```python
from build123d import *

# Parameters (mm, degrees)
PCB_DEPTH           = 1.56
ESQUISSE2_W         = 6
ESQUISSE2_H         = 6
ESQUISSE2_R         = 1.75
CORPSBP_DEPTH       = 3.52
ESQUISSE2_3_R       = 1.75
BPBP_DEPTH          = 4.32
ESQUISSE2_4_W       = 3.54
ESQUISSE2_4_H       = 8.6
CORPSONOFF_DEPTH    = 3.5
ESQUISSE2_5_W       = 1.5
ESQUISSE2_5_H       = 3.6
BPONOFF_DEPTH       = 5.5
ESQUISSE2_6_W       = 5
ESQUISSE2_6_H       = 5
BOSS_EXTRU_9_DEPTH  = 1.5
ESQUISSE5_R         = 5.9
BUZZER_DEPTH        = 9.9
ESQUISSE5_4_W       = 7.74
ESQUISSE5_4_H       = 5
ISP_DEPTH           = 8.6
CR2032_DEPTH        = 7
ESQUISSE6_W         = 4
ESQUISSE6_H         = 4
BOSS_EXTRU_10_DEPTH = 1.5


with BuildPart() as part:
    # Esquisse1 → PCB (new body)
    with BuildSketch(Plane.XY):
        with BuildLine():
            Line((-25.15, -25.15), (25.15, -25.15))
            ThreePointArc((25.15, -25.15), (28.685533906, -23.685533906), (30.15, -20.15))
            Line((30.15, -20.15), (30.15, 20.15))
            ThreePointArc((30.15, 20.15), (28.685533906, 23.685533906), (25.15, 25.15))
            Line((25.15, 25.15), (-25.15, 25.15))
            ThreePointArc((-25.15, 25.15), (-28.685533906, 23.685533906), (-30.15, 20.15))
            Line((-30.15, 20.15), (-30.15, -20.15))
            ThreePointArc((-30.15, -20.15), (-28.685533906, -23.685533906), (-25.15, -25.15))
        make_face()
    extrude(amount=PCB_DEPTH)

    # Esquisse2 → CorpsBp (add)
    # profile 1 of 8: a face of its own
    with BuildSketch(Plane.XY.offset(1.56)):
        with Locations((-20.15, 9.75)):
            Rectangle(ESQUISSE2_W, ESQUISSE2_H)
        with Locations((-20.15, 9.75)):
            Circle(ESQUISSE2_R, mode=Mode.SUBTRACT)
    # profile 2 of 8: a face of its own
    with BuildSketch(Plane.XY.offset(1.56)):
        with Locations((-20.45, -10.35)):
            Rectangle(ESQUISSE2_W, ESQUISSE2_H)
        with Locations((-20.45, -10.35)):
            Circle(ESQUISSE2_R, mode=Mode.SUBTRACT)
    # profile 3 of 8: a face of its own
    with BuildSketch(Plane.XY.offset(1.56)):
        with Locations((20.31, 9.55)):
            Rectangle(ESQUISSE2_W, ESQUISSE2_H)
        with Locations((20.31, 9.55)):
            Circle(ESQUISSE2_R, mode=Mode.SUBTRACT)
    # profile 4 of 8: a face of its own
    with BuildSketch(Plane.XY.offset(1.56)):
        with Locations((19.85, -10.35)):
            Rectangle(ESQUISSE2_W, ESQUISSE2_H)
        with Locations((19.85, -10.35)):
            Circle(ESQUISSE2_R, mode=Mode.SUBTRACT)
    # profile 5 of 8: a face of its own
    with BuildSketch(Plane.XY.offset(1.56)):
        with Locations((-20.45, -10.35)):
            Circle(ESQUISSE2_R)
    # profile 6 of 8: a face of its own
    with BuildSketch(Plane.XY.offset(1.56)):
        with Locations((-20.15, 9.75)):
            Circle(ESQUISSE2_R)
    # profile 7 of 8: a face of its own
    with BuildSketch(Plane.XY.offset(1.56)):
        with Locations((20.31, 9.55)):
            Circle(ESQUISSE2_R)
    # profile 8 of 8: a face of its own
    with BuildSketch(Plane.XY.offset(1.56)):
        with Locations((19.85, -10.35)):
            Circle(ESQUISSE2_R)
    extrude(amount=CORPSBP_DEPTH)

    # Esquisse2_3 → BpBp (add)
    with BuildSketch(Plane.XY.offset(1.56)):
        with Locations((20.31, 9.55)):
            Circle(ESQUISSE2_3_R)
        with Locations((-20.15, 9.75)):
            Circle(ESQUISSE2_3_R)
        with Locations((-20.45, -10.35)):
            Circle(ESQUISSE2_3_R)
        with Locations((19.85, -10.35)):
            Circle(ESQUISSE2_3_R)
    extrude(amount=BPBP_DEPTH)

    # Esquisse2_4 → CorpsOnOff (add)
    with BuildSketch(Plane.XY.offset(1.56)):
        with Locations((9.04, 9.85)):
            Rectangle(ESQUISSE2_4_W, ESQUISSE2_4_H)
    extrude(amount=CORPSONOFF_DEPTH)

    # Esquisse2_5 → BpOnOff (add)
    with BuildSketch(Plane.XY.offset(1.56)):
        with Locations((9.04, 9.85)):
            Rectangle(ESQUISSE2_5_W, ESQUISSE2_5_H)
    extrude(amount=BPONOFF_DEPTH)

    # Esquisse2_6 → Boss.-Extru.9 (add)
    with BuildSketch(Plane.XY.offset(1.56)):
        with Locations((-12.5, 17.5)):
            Rectangle(ESQUISSE2_6_W, ESQUISSE2_6_H)
        with Locations((-12.5, -17.5)):
            Rectangle(ESQUISSE2_6_W, ESQUISSE2_6_H)
        with Locations((12.5, -17.5)):
            Rectangle(ESQUISSE2_6_W, ESQUISSE2_6_H)
        with Locations((12.5, 17.5)):
            Rectangle(ESQUISSE2_6_W, ESQUISSE2_6_H)
    extrude(amount=BOSS_EXTRU_9_DEPTH)

    # Esquisse5 → Buzzer (add)
    with BuildSketch(Plane(origin=(0, 0, 0), x_dir=(-1, 0, 0), z_dir=(0, 0, -1))):
        with Locations(Location((0.75, -18.69, 0), (0, 0, 180))):
            Circle(ESQUISSE5_R)
    extrude(amount=BUZZER_DEPTH)

    # Esquisse5_4 → ISP (add)
    with BuildSketch(Plane(origin=(0, 0, 0), x_dir=(-1, 0, 0), z_dir=(0, 0, -1))):
        with Locations((0, 16.45)):
            Rectangle(ESQUISSE5_4_W, ESQUISSE5_4_H)
    extrude(amount=ISP_DEPTH)

    # Esquisse5_5 → CR2032 (add)
    with BuildSketch(Plane(origin=(0, 0, 0), x_dir=(-1, 0, 0), z_dir=(0, 0, -1))):
        with BuildLine():
            Line((9.061920088, 3.25), (15.15, 3.25))
            Line((15.15, 3.25), (15.15, -3.35))
            Line((15.15, -3.35), (9.061920088, -3.35))
            ThreePointArc((9.061920088, -3.35), (-13.25, -0.05), (9.061920088, 3.25))
        make_face()
    extrude(amount=CR2032_DEPTH)

    # Esquisse6 → Boss.-Extru.10 (add)
    with BuildSketch(Plane.XY.offset(1.56)):
        with Locations((-24.35, -17.8)):
            Rectangle(ESQUISSE6_W, ESQUISSE6_H)
    extrude(amount=BOSS_EXTRU_10_DEPTH)


solid = part.part
```
CAD build for the part. Positions are in the model's coordinates, mm. A direction names the side the tool comes from. Round coordinates to 2 decimals unless told otherwise and drop trailing zeros. Write each loop counter-clockwise with the first axis right and the second up, starting at its lowest first coordinate (ties: lowest second). Pieces come first, ordered by that corner, then holes. Notation, with made-up numbers: (-36, 83.25) - (23, 83.25) arc R25 ccw to (23, 106.25) - close; hole circle Ø10 at (88.5, -31.75). An arc over 180 degrees is marked (long way). Return JSON: item names as keys, results as strings. Group by question number.
Item 1: Band-saw the part on B-B on z = -6. List the corners of the cut face in (x, y).
Item 2: Band-saw the part on A-A on x = -11.5. List the corners of the cut face in (y, z).
Item 3: Band-saw the part on C-C on y = -18.69. List the corners of the cut face in (x, z).
Item 4: Probe probe 1 along Y at (x, z) = (-10.5, 2.75); probe 2 along X at (y, z) = (-15.5, 2.25); probe 3 along Z at (x, y) = (4, -2). List the from-to ranges inside material, lowest first.
Item 5: Flat gauge pins, fed straight in: pin 1 Ø3 at (x, y) = (-19.5, 10.5) entering from +Z; pin 2 Ø0.6 at (y, z) = (10, 6.5) entering from -X; pin 3 Ø8 at (y, z) = (16, 4) entering from +X; pin 4 Ø1 at (x, y) = (-9, 19) entering from -Z. Where does each tip first touch, or does it go through?
Item 6: 3-axis set-ups, long thin cutter, end or side, ignore diameter. For faces 1 (the face through (12, 15, 2)), 2 (the face through (10, 17, 2)), 3 (the face through (12, 18, 3.06)), 4 (the face through (-26.35, -18, 2)): which of +Z, -Z, +X, -X, +Y, -Y reach the whole face in a straight line?
Item 7: Band-saw the part on D-D on y = 18. List the corners of the cut face in (x, z), plus the area to 3 significant figures.
Item 8: Mould opens along Y. For faces 5 (the face through (21, -12, 5.08)), 6 (the face through (10, 10, 5.06)), 7 (the face through (28.65, -23.72, 0.77)) say: +Y half, -Y half, draft (parallel to the pull), parting line (faces both ways), or undercut.
Resolved:
{
 "1": {"outline": "(-15.15, -3.35) - (-9.06, -3.35) arc R11.4 ccw (long way) to (-9.06, 3.25) - (-15.15, 3.25) - close; circle Ø11.8 at (-0.75, -18.69); (-3.87, 13.95) - (3.87, 13.95) - (3.87, 18.95) - (-3.87, 18.95) - close"},
 "2": {"outline": "(-25.15, 0) - (-3.35, 0) - (-3.35, -7) - (3.25, -7) - (3.25, 0) - (25.15, 0) - (25.15, 1.56) - (20, 1.56) - (20, 3.06) - (15, 3.06) - (15, 1.56) - (-15, 1.56) - (-15, 3.06) - (-20, 3.06) - (-20, 1.56) - (-25.15, 1.56) - close"},
 "3": {"outline": "(-30.15, 0) - (-6.65, 0) - (-6.65, -9.9) - (5.15, -9.9) - (5.15, 0) - (30.15, 0) - (30.15, 1.56) - (15, 1.56) - (15, 3.06) - (10, 3.06) - (10, 1.56) - (-10, 1.56) - (-10, 3.06) - (-15, 3.06) - (-15, 1.56) - (-22.35, 1.56) - (-22.35, 3.06) - (-26.35, 3.06) - (-26.35, 1.56) - (-30.15, 1.56) - close"},
 "4": {"probe 1": "y = -20 to -15, 15 to 20", "probe 2": "x = -15 to -10, 10 to 15", "probe 3": "z = -7 to 1.56"},
 "5": {"pin 1": "stops at z = 5.88", "pin 2": "stops at x = 8.29", "pin 3": "stops at x = 30.15", "pin 4": "stops at z = 0"},
 "6": {"face 1": "+Z, +X, -X", "face 2": "+Z, +Y", "face 3": "+Z, +X, -X, +Y", "face 4": "+Z, -X, +Y, -Y"},
 "7": {"outline": "(-30.15, 0) - (-3.87, 0) - (-3.87, -8.6) - (3.87, -8.6) - (3.87, 0) - (30.15, 0) - (30.15, 1.56) - (15, 1.56) - (15, 3.06) - (10, 3.06) - (10, 1.56) - (-10, 1.56) - (-10, 3.06) - (-15, 3.06) - (-15, 1.56) - (-30.15, 1.56) - close", "area": "176 mm²"},
 "8": {"face 5": "undercut", "face 6": "draft", "face 7": "-Y half"}
}
